Geometry: final body of the model. Coordinates: model frame, mm. A direction names the side the tool comes from. Coordinates: 2 decimals unless noted, no trailing zeros. Order: outer loops, then holes, each group sorted by start corner. A loop starts at its lowest first (then second) coordinate and runs counter-clockwise, first axis right, second up. Notation, with made-up numbers: M -22,69.5 L -7,69.5 A22 cw -7,107.5 Z; hole C 25,52 d5. An arc over 180 degrees is marked long. One line per question, with ' | ' between items.
from build123d import *

# Parameters (mm, degrees)
SKETCH_W        = 100
SKETCH_H        = 64
SKETCH_R        = 5
SKETCH_R_2      = 3.2
SKETCH_R_3      = 4
PAD_DEPTH       = 15
SKETCH001_R     = 11.02
POCKET_DEPTH    = 7.2
SKETCH002_R     = 6
POCKET001_DEPTH = 6
SKETCH003_R     = 3.2
POCKET002_DEPTH = 15
SKETCH004_R     = 8.4
POCKET003_DEPTH = 8


with BuildPart() as part:
    # Sketch → Pad (new body)
    with BuildSketch(Plane.XY):
        with Locations((50, 32)):
            Rectangle(SKETCH_W, SKETCH_H)
        with Locations((50, 42.85)):
            Circle(SKETCH_R, mode=Mode.SUBTRACT)
        with Locations((20, 10)):
            Circle(SKETCH_R_2, mode=Mode.SUBTRACT)
        with Locations((80, 10)):
            Circle(SKETCH_R_2, mode=Mode.SUBTRACT)
        with Locations((82, 42.85)):
            Circle(SKETCH_R_3, mode=Mode.SUBTRACT)
        with Locations((18, 42.85)):
            Circle(SKETCH_R_3, mode=Mode.SUBTRACT)
    extrude(amount=PAD_DEPTH)

    # Sketch001 (on Face11 of Pad) → Pocket (cut)
    with BuildSketch(Plane.XY.offset(15)):
        with Locations((50, 42.85)):
            Circle(SKETCH001_R)
    extrude(amount=-POCKET_DEPTH, mode=Mode.SUBTRACT)

    # Sketch002 (on Face4 of Pocket) → Pocket001 (cut)
    with BuildSketch(Plane(origin=(0, 0, 0), x_dir=(1, 0, 0), z_dir=(0, 0, -1))):
        with Locations((20, -10)):
            Circle(SKETCH002_R)
        with Locations((80, -10)):
            Circle(SKETCH002_R)
        with Locations((40, -10)):
            Circle(SKETCH002_R)
        with Locations((60, -10)):
            Circle(SKETCH002_R)
    extrude(amount=-POCKET001_DEPTH, mode=Mode.SUBTRACT)

    # Sketch003 (on Face5 of Pocket001) → Pocket002 (cut)
    with BuildSketch(Plane.XY.offset(15)):
        with Locations((40, 10)):
            Circle(SKETCH003_R)
        with Locations((60, 10)):
            Circle(SKETCH003_R)
    extrude(amount=-POCKET002_DEPTH, mode=Mode.SUBTRACT)

    # Sketch004 (on Face4 of Pocket002) → Pocket003 (cut)
    with BuildSketch(Plane(origin=(0, 0, 0), x_dir=(1, 0, 0), z_dir=(0, 0, -1))):
        with Locations((18, -42.85)):
            Circle(SKETCH004_R)
        with Locations((82, -42.85)):
            Circle(SKETCH004_R)
    extrude(amount=-POCKET003_DEPTH, mode=Mode.SUBTRACT)


solid = part.part
1. Section C-C, the plane x = 18. Output: boundary loops of the cut face in (y, z), and give its area (3 significant figures).
Response values:
outline: M 0,0 L 4.34,0 L 4.34,6 L 7.5,6 L 7.5,15 L 0,15 Z; M 12.5,6 L 15.66,6 L 15.66,0 L 34.45,0 L 34.45,8 L 38.85,8 L 38.85,15 L 12.5,15 Z; M 46.85,8 L 51.25,8 L 51.25,0 L 64,0 L 64,15 L 46.85,15 Z | area: 657 mm^2
2. Access query for faces 4 (the face through (38.99, 43.33, 11.45)), 5 (the face through (81.479, 46.816, 11.451)), 6 (the face through (43, 13, 6)). Directions: +Z, -Z, +X, -X, +Y, -Y. A direction counts if a zero-diameter tool reaches every point of the face in a straight line with its end or side. Return the directions, or none.
Response values:
face 4: +Z | face 5: +Z, -Z | face 6: -Z
3. Section B-B, the plane x = 50. Output: boundary loops of the cut face in (y, z), and give its area (3 significant figures).
Response values:
outline: M 0,0 L 37.85,0 L 37.85,7.8 L 31.83,7.8 L 31.83,15 L 0,15 Z; M 47.85,0 L 64,0 L 64,15 L 53.87,15 L 53.87,7.8 L 47.85,7.8 Z | area: 723 mm^2
4. Draft query along X for faces 1 (the face through (86, 45, 8)), 2 (the face through (49, 0, 7)), 3 (the face through (16.91, 34.52, 3.94)). Return one class per face: pulls with the +X half, pulls with the -X half, needs draft (parallel to the pull), parting line crosses it, or undercut.
Response values:
face 1: undercut | face 2: needs draft | face 3: undercut
5. Section A-A, the plane y = 42.85. Output: boundary loops of the cut face in (x, z).
Response values:
outline: M 0,0 L 9.6,0 L 9.6,8 L 14,8 L 14,15 L 0,15 Z; M 22,8 L 26.4,8 L 26.4,0 L 45,0 L 45,7.8 L 38.98,7.8 L 38.98,15 L 22,15 Z; M 55,0 L 73.6,0 L 73.6,8 L 78,8 L 78,15 L 61.02,15 L 61.02,7.8 L 55,7.8 Z; M 86,8 L 90.4,8 L 90.4,0 L 100,0 L 100,15 L 86,15 Z
6. Material intervals for line 1 (X direction, y = 10, z = 2.5); line 2 (X direction, y = 13, z = 3.5); line 3 (Y direction, x = 80, z = 12.25), sorted ascending. Write a range as [from, to].
Response values:
line 1: x = [0, 14], [26, 34], [46, 54], [66, 74], [86, 100] | line 2: x = [0, 14.8], [25.2, 34.8], [45.2, 54.8], [65.2, 74.8], [85.2, 100] | line 3: y = [0, 6.8], [13.2, 39.39], [46.31, 64]
7. Section D-D, the plane x = 80. Output: boundary loops of the cut face in (y, z).
Response values:
outline: M 0,0 L 4,0 L 4,6 L 6.8,6 L 6.8,15 L 0,15 Z; M 13.2,6 L 16,6 L 16,0 L 34.69,0 L 34.69,8 L 39.39,8 L 39.39,15 L 13.2,15 Z; M 46.31,8 L 51.01,8 L 51.01,0 L 64,0 L 64,15 L 46.31,15 Z
8. Pin query (flat end, axial travel): P1, Ø6, axis at x = 20, y = 10, coming from the +Z side; P2, Ø11, axis at x = 40, y = 10, coming from the -Z side; P3, Ø1, axis at x = 86, y = 41.5, coming from the -Z side. Return the tip coordinate at first contact, or that it passes through.
Response values:
P1: passes through | P2: stops at z = 6 | P3: stops at z = 8
